```python
from build123d import *

# Parameters (mm, degrees)
SKETCH1_R           = 8.5
SKETCH1_R_2         = 4
BOSS_EXTRUDE1_DEPTH = 4.2
CHAMFER1_SIZE       = 0.3
FILLET1_R           = 0.2


with BuildPart() as part:
    # Sketch1 → Boss-Extrude1 (new body)
    with BuildSketch(Plane.XY):
        Circle(SKETCH1_R)
        Circle(SKETCH1_R_2, mode=Mode.SUBTRACT)
    extrude(amount=BOSS_EXTRUDE1_DEPTH)

    # Chamfer1
    chamfer1_edges = [part.edges().sort_by_distance(p)[0] for p in [
        (-4, 0, 0),
        (-4, 0, 4.2),
    ]]
    chamfer(chamfer1_edges, length=CHAMFER1_SIZE)

    # Fillet1
    fillet1_edges = [part.edges().sort_by_distance(p)[0] for p in [
        (-8.5, 0, 0),
        (-8.5, 0, 4.2),
    ]]
    fillet(fillet1_edges, radius=FILLET1_R)


solid = part.part
```
For this review, take the finished solid that the model builds, in its own axes (mm). Round coordinates to 2 decimals unless told otherwise and drop trailing zeros. Loops run counter-clockwise (first coordinate to the right, second up) from the corner with the lowest first, then second, coordinate; pieces in that order, holes last.
Q1. Add section A-A on x = 0. Write out the cut boundary in (y, z), plus the area to 3 significant figures.
Result sheet:
outline: (-8.5, 0.2) arc R0.2 ccw to (-8.3, 0) - (-4.3, 0) - (-4, 0.3) - (-4, 3.9) - (-4.3, 4.2) - (-8.3, 4.2) arc R0.2 ccw to (-8.5, 4) - close; (4, 0.3) - (4.3, 0) - (8.3, 0) arc R0.2 ccw to (8.5, 0.2) - (8.5, 4) arc R0.2 ccw to (8.3, 4.2) - (4.3, 4.2) - (4, 3.9) - close
area: 37.6 mm2
Q2. Mouldability with a two-part tool opening along X and no side actions: class faces 1 (the face through (4.57, 7.167, 2.073)), 2 (the face through (4, -4, 4.2)), 3 (the face through (-0.867, -3.905, 2.075)) as +X half, -X half, draft (parallel to the pull), parting line (faces both ways), or undercut.
Result sheet:
face 1: parting line
face 2: draft
face 3: undercut
Q3. To check wall thickness, follow line 1 along Y through (x, z) = (0, 2.4); line 2 along X through (y, z) = (-2.25, 0.8); line 3 along Y through (x, z) = (-1.75, 3.3). State the ranges of each line that lie inside material, in increasing order.
Result sheet:
line 1: y = -8.5 to -4, 4 to 8.5
line 2: x = -8.2 to -3.31, 3.31 to 8.2
line 3: y = -8.32 to -3.6, 3.6 to 8.32
Q4. Add section C-C on z = 3.35. Write out the cut boundary in (x, y), plus the area to 3 significant figures.
Result sheet:
outline: circle Ø17 at (0, 0); hole circle Ø8 at (0, 0)
area: 177 mm2
Q5. Insertion check: pin 1 Ø6.5 at (x, y) = (0, 0) entering from -Z; pin 2 Ø2 at (x, z) = (-2.5, 2) entering from +Y; pin 3 Ø1 at (x, y) = (-1.5, 4) entering from -Z; pin 4 Ø2 at (x, z) = (-6.5, 2) entering from +Y. Each pin has a flat end and moves straight along its axis. Give the tip position at first contact, or say it passes through.
Result sheet:
pin 1: passes through
pin 2: stops at y = 8.37
pin 3: stops at z = 0
pin 4: stops at y = 6.48
